Autodesk Inventor part; units mm, degrees
ref_plane "YZ Plane" through (0, 0, 0) normal (1, 0, 0) x (0, 1, 0)
ref_plane "XZ Plane" through (0, 0, 0) normal (0, 1, 0) x (-1, 0, 0)
ref_plane "XY Plane" through (0, 0, 0) normal (0, 0, 1) x (1, 0, 0)
sketch "Sketch1" plane through (0, 0, 0) normal (0, 0, 1) x (1, 0, 0)
  line L0 (0, 0) -> (15, 0)
  line L1 (15, 0) -> (15, 15)
  line L2 (15, 15) -> (0, 15)
  line L3 (0, 15) -> (0, 0)
  dimension "d0" = 15
  dimension "d1" = 15
extrude "Extrusion1" add sketch "Sketch1" against normal blind 4
sketch "Sketch2" plane through (0, 0, -4) normal (0, 0, -1) x (-1, 0, 0)
  circle A0 centre (-7.5, 7.5) radius 7.5
  point P0 (0, 0)
  dimension "d4" = 15
extrude "Extrusion2" add sketch "Sketch2" along normal blind 3
sketch "Sketch3" plane through (7.5, 7.5, -7) normal (0, 0, -1) x (-1, 0, 0)
  circle A0 centre (0, 0) radius 1
  point P0 (7.5, -7.5)
  dimension "d7" = 2
extrude "Extrusion3" add sketch "Sketch3" along normal blind 7
sketch "Sketch4" plane through (0, 0, 0) normal (0, 0, 1) x (1, 0, 0)
  line L0 (0.2915, 14.885) -> (14.8969, 14.885) construction
  line L1 (14.8969, 14.885) -> (14.8969, 0.1242) construction
  line L2 (14.8969, 0.1242) -> (0.2915, 0.1242) construction
  line L3 (0.2915, 0.1242) -> (0.2915, 14.885) construction
  point P0 (0, 0)
sketch "Sketch5" plane through (0, 0, 0) normal (0, -1, 0) x (1, 0, 0)
  line L0 (0.1529, -0.1223) -> (14.8622, -0.1223) construction
  line L1 (14.8622, -0.1223) -> (14.8622, -3.792) construction
  line L2 (14.8622, -3.792) -> (0.1529, -3.792) construction
  line L3 (0.1529, -3.792) -> (0.1529, -0.1223) construction
  point P0 (0, 0)
properties part number "Input Motor" material "ABS Plastic"
Geometry check sheet. Reference: the model listing, model coordinates, mm. A direction names the side the tool comes from. Round coordinates to 2 decimals unless told otherwise and drop trailing zeros. Order: outer loops, then holes, each group sorted by start corner. A loop starts at its lowest first (then second) coordinate and runs counter-clockwise, first axis right, second up. Notation, with made-up numbers: M -23,81.5 L 13,81.5 A12 ccw 13,98.5 Z; hole C 81,78 d1. An arc over 180 degrees is marked long. Answer in a Markdown table with one row per item.
(1) Sectioned sample at A-A, the plane x = 2.75. Record the cut outline in (y, z).
Responses:
| item | result |
|---|---|
| outline | M 0,-4 L 1.7,-4 L 1.7,-7 L 13.3,-7 L 13.3,-4 L 15,-4 L 15,0 L 0,0 Z |
(2) Scan lines: probe 1 along Z at (x, y) = (2.25, 9.25); probe 2 along Z at (x, y) = (14.25, 11.5); probe 3 along X at (y, z) = (4.25, -5.5). Record each from-to range of solid material in increasing order. Write a range as from..to.
Responses:
| item | result |
|---|---|
| probe 1 | z = -7..0 |
| probe 2 | z = -4..0 |
| probe 3 | x = 0.74..14.26 |
(3) Sectioned sample at C-C, the plane z = -6.75. Record the cut outline in (x, y), and give its area (3 significant figures).
Responses:
| item | result |
|---|---|
| outline | C 7.5,7.5 d15 |
| area | 177 mm² |
(4) Tool access check on faces 1 (the face through (2, 2, -4)), 2 (the face through (13, 13, -4)), 3 (the face through (13, 2, -4)), 4 (the face through (13, 2.4, -5.5)). Record the directions out of +Z, -Z, +X, -X, +Y, -Y that give a thin tool (end or side, any length) a straight path to the whole face; none if there is none.
Responses:
| item | result |
|---|---|
| face 1 | -Z, -X, -Y |
| face 2 | -Z, +X, +Y |
| face 3 | -Z, +X, -Y |
| face 4 | -Z |
(5) Sectioned sample at D-D, the plane z = -10.25. Record the cut outline in (x, y).
Responses:
| item | result |
|---|---|
| outline | C 7.5,7.5 d2 |
(6) Sectioned sample at B-B, the plane y = 5.5. Record the cut outline in (x, z), and give its area (3 significant figures).
Responses:
| item | result |
|---|---|
| outline | M 0,-4 L 0.27,-4 L 0.27,-7 L 14.73,-7 L 14.73,-4 L 15,-4 L 15,0 L 0,0 Z |
| area | 103 mm² |
(7) Go/stop test with flat-tipped pins: P1, Ø1.5, axis at y = 11, z = -4.5, coming from the +X side; P2, Ø4, axis at x = 11, y = 11.5, coming from the -Z side; P3, Ø1.5, axis at y = 11, z = -12, coming from the -X side; P4, Ø2, axis at x = 6, z = -10.5, coming from the -Y side. Record where each tip stops, or that it passes through.
Responses:
| item | result |
|---|---|
| P1 | stops at x = 15 |
| P2 | stops at z = -7 |
| P3 | passes through |
| P4 | stops at y = 6.63 |
